from build123d import *

# Parameters (mm, degrees)
KRUHOV_POLE1_COUNT = 7


with BuildPart() as part:
    # Skica1 → Rotovat1 (revolve)
    with BuildSketch(Plane.XY, mode=Mode.PRIVATE) as rotovat1_sk:
        with BuildLine():
            Line((-80, 2.5), (-61.443375673, 2.5))
            Line((-61.443375673, 2.5), (-60, 0))
            Line((-60, 0), (80, 0))
            Line((80, 0), (80, 7.5))
            Line((80, 7.5), (63, 7.5))
            Line((63, 7.5), (63, 10))
            Line((63, 10), (50, 10))
            Line((50, 10), (50, 13))
            Line((50, 13), (2.414213562, 13))
            Line((2.414213562, 13), (1.707106781, 12.292893219))
            ThreePointArc((1.707106781, 12.292893219), (0.617316568, 12.076120467), (0, 13))
            Line((0, 13), (0, 15))
            Line((0, 15), (-20, 15))
            Line((-20, 15), (-25.196152423, 12))
            Line((-25.196152423, 12), (-79, 12))
            Line((-79, 12), (-80, 11))
            Line((-80, 11), (-80, 2.5))
        make_face()
    revolve(rotovat1_sk.sketch.rotate(Axis((89.49015633, 0, 0), (-1, 0, 0)), 90), axis=Axis((89.49015633, 0, 0), (-1, 0, 0)))  # turned: the seam where the file's is

    # Odebrat tažením po křivce1: sweep along a path in Skica2
    with BuildLine(Plane.XY) as odebrat_ta_en_m_po_k_ivce1_path:
        Line((-80, 9), (-40, 9))
        ThreePointArc((-40, 9), (-30.024182748, 11.665552499), (-22.707471957, 18.951692985))
    # Skica3 → Odebrat tažením po křivce1 (sweep, cut)
    with BuildSketch(Plane.ZY.offset(80)):
        Polygon((-4.16819533, 13.621449875), (-1.5, 9), (1.5, 9), (4.16819533, 13.621449875), align=None)
    odebrat_ta_en_m_po_k_ivce1 = sweep(path=odebrat_ta_en_m_po_k_ivce1_path.line, mode=Mode.SUBTRACT)

    # Kruhové pole1: Odebrat tažením po křivce1 ×7 about axis
    kruhov_pole1_axis = Axis((0, 0, 0), (1, 0, 0))
    for i in range(1, KRUHOV_POLE1_COUNT):
        add(odebrat_ta_en_m_po_k_ivce1.rotate(kruhov_pole1_axis, i * 360 / KRUHOV_POLE1_COUNT), mode=Mode.SUBTRACT)


solid = part.part
The model under review builds one solid part; all positions refer to its coordinate system, in mm. A direction names the side the tool comes from. Give positions to 0.01 mm unless a question says otherwise; leave off trailing zeros. Loops run counter-clockwise (first coordinate to the right, second up) from the corner with the lowest first, then second, coordinate; pieces in that order, holes last. Notation, with made-up numbers: (46, -4.75) -> (72, -4.75) arc R18 cw to (72, 24.25) -> close; hole circle Ø4 at (57, 39.25). An arc over 180 degrees is marked (long way). Answer as a JSON object with one key per item and string values. Group by question number.
Q1. Take a section at B-B (x = 39.5). Write out the cut boundary in (y, z).
Q2. Take a section at A-A (x = -54). Write out the cut boundary in (y, z).
Q3. Draft analysis for pull direction Z (two halves, no side actions). For faces 1 (the flat face through (-59.72, -1.98, 8.78)), 2 (the flat face through (-59.72, 8.171, -6.645)), 3 (the conical face through (-36.13, -8.66, 6.66)), state which applies: pulls with the +Z half, pulls with the -Z half, needs draft (parallel to the pull), parting line crosses it, or undercut.
Q4. Tool access review of faces 4 (the flat face through (50, 8, 7)), 5 (the conical face through (-36.14, -4.6, 9.96)), 6 (the conical face through (-36.14, 4.92, 9.8)), 7 (the conical face through (-36.13, -4.57, -9.93)): name each direction out of +Z, -Z, +X, -X, +Y, -Y from which nothing blocks a thin tool from reaching the whole face with its end or side.
Q5. Take a section at C-C (x = -15.5). Write out the cut boundary in (y, z), plus the area to 3 significant figures.
Q6. Insertion check: pin 1 (8 mm diameter, centred on y = 12, z = 11.5, fed in from +X); pin 2 (4 mm diameter, centred on x = -14.5, z = 5, fed in from +Y); pin 3 (1.5 mm diameter, centred on x = 61, y = 5, fed in from +Z); pin 4 (12 mm diameter, centred on y = 7.5, z = 11.5, fed in from -X). Each pin has a flat end and moves straight along its axis. Give the tip position at first contact, or say it passes through.
Q7. Wall thickness on line 1 along Y through (x, z) = (-67.5, 0); line 2 along X through (y, z) = (6.25, -4.75); line 3 along Z through (x, y) = (-46, 9.75): over which ranges is each line inside the solid? List them lowest first.
Answer below:
{
 "1": {"outline": "circle Ø26 at (0, 0)"},
 "2": {"outline": "(-11.77, -2.33) -> (-8.76, -2.55) -> (-7.46, -5.26) -> (-9.16, -7.75) arc R12 ccw to (-5.52, -10.66) -> (-3.47, -8.44) -> (-0.54, -9.11) -> (0.35, -11.99) arc R12 ccw to (4.89, -10.96) -> (4.44, -7.97) -> (6.78, -6.1) -> (9.6, -7.2) arc R12 ccw to (11.62, -3.01) -> (9, -1.5) -> (9, 1.5) -> (11.62, 3.01) arc R12 ccw to (9.6, 7.2) -> (6.78, 6.1) -> (4.44, 7.97) -> (4.89, 10.96) arc R12 ccw to (0.35, 11.99) -> (-0.54, 9.11) -> (-3.47, 8.44) -> (-5.52, 10.66) arc R12 ccw to (-9.16, 7.75) -> (-7.46, 5.26) -> (-8.76, 2.55) -> (-11.77, 2.33) arc R12 ccw to start"},
 "3": {"face 1": "pulls with the +Z half", "face 2": "pulls with the -Z half", "face 3": "undercut"},
 "4": {"face 4": "+X", "face 5": "+Z, -X", "face 6": "-X, +Y", "face 7": "-Z, -X"},
 "5": {"outline": "circle Ø30 at (0, 0)", "area": "707 mm2"},
 "6": {"pin 1": "stops at x = 50", "pin 2": "stops at y = 14.7", "pin 3": "stops at z = 9.05", "pin 4": "stops at x = -80"},
 "7": {"line 1": "y = -12 to -2.5, 2.5 to 9", "line 2": "x = -80 to 63", "line 3": "z = -7 to -1.93, 1.93 to 7"}
}
